Geometry: final body of the model. Coordinates: model frame, mm. A direction names the side the tool comes from. Round coordinates to 2 decimals unless told otherwise and drop trailing zeros. Order: outer loops, then holes, each group sorted by start corner. A loop starts at its lowest first (then second) coordinate and runs counter-clockwise, first axis right, second up. Notation, with made-up numbers: M 89.25,0 L 126.25,0 A22 cw 126.25,10 Z; hole C 46.25,60.25 d11. An arc over 180 degrees is marked long. Return JSON: item names as keys, results as strings. Group by question number.
Q1. Cut plane A-A on x = 25. Output: boundary loops of the cut face in (y, z).
Q2. Cut plane D-D on z = 5. Output: boundary loops of the cut face in (x, y).
Q3. Ray query, probe 1 along Y at (x, z) = (25, -0.8); probe 2 along Z at (x, y) = (6, 42.5); probe 3 along Y at (x, z) = (9.5, 5.5). Return the intervals inside material, ascending.
Q4. Mould query, pull axis Y, two halves, no side actions, for faces 3 (the face through (26.301, 24.143, -0.986)), 4 (the face through (25, 45, -1)), 5 (the face through (0, 1, 13)). Classes: released by +Y, released by -Y, zero draft, split by the parting line, or undercut.
Q5. Cut plane B-B on y = 30. Output: boundary loops of the cut face in (x, z).
Q6. Cut plane C-C on x = 44. Output: boundary loops of the cut face in (y, z), and give its area (3 significant figures).
Q7. Contact query for flat-ended pins moving along their axis: pin 1 (15 mm diameter, centred on x = 14, z = 16.5, fed in from +Y); pin 2 (1.5 mm diameter, centred on x = 41, y = 36.5, fed in from +Z). Output: stop coordinate, or through.
Q8. Access query for faces 1 (the face through (25, 23, -2)), 2 (the face through (25, 2, 25)). Directions: +Z, -Z, +X, -X, +Y, -Y. A direction counts if a zero-diameter tool reaches every point of the face in a straight line with its end or side. Return the directions, or none.
```python
from build123d import *

# Parameters (mm, degrees)
SKETCH1_W           = 50
SKETCH1_H           = 50
BOSS_EXTRUDE1_DEPTH = 2
SKETCH2_W           = 50
SKETCH2_H           = 45
SKETCH2_R           = 6
BOSS_EXTRUDE2_DEPTH = 2


with BuildPart() as part:
    # Sketch1 → Boss-Extrude1 (new body)
    with BuildSketch(Plane(origin=(0, 0, 0), x_dir=(1, 0, 0), z_dir=(0, 1, 0))):
        with Locations((25, -25)):
            Rectangle(SKETCH1_W, SKETCH1_H)
    extrude(amount=BOSS_EXTRUDE1_DEPTH)

    # Sketch2 → Boss-Extrude2 (add)
    with BuildSketch(Plane(origin=(0, 0, 0), x_dir=(-1, 0, 0), z_dir=(0, 0, -1))):
        with Locations((-25, 22.5)):
            Rectangle(SKETCH2_W, SKETCH2_H)
        with Locations((-25, 30)):
            Circle(SKETCH2_R, mode=Mode.SUBTRACT)
    extrude(amount=BOSS_EXTRUDE2_DEPTH)


solid = part.part
```
Result sheet:
{
 "1": {"outline": "M 0,-2 L 24,-2 L 24,0 L 2,0 L 2,50 L 0,50 Z; M 36,-2 L 45,-2 L 45,0 L 36,0 Z"},
 "2": {"outline": "M 0,0 L 50,0 L 50,2 L 0,2 Z"},
 "3": {"probe 1": "y = 0 to 24, 36 to 45", "probe 2": "z = -2 to 0", "probe 3": "y = 0 to 2"},
 "4": {"face 3": "undercut", "face 4": "released by +Y", "face 5": "zero draft"},
 "5": {"outline": "M 0,-2 L 19,-2 L 19,0 L 0,0 Z; M 31,-2 L 50,-2 L 50,0 L 31,0 Z"},
 "6": {"outline": "M 0,-2 L 45,-2 L 45,0 L 2,0 L 2,50 L 0,50 Z", "area": "190 mm²"},
 "7": {"pin 1": "stops at y = 2", "pin 2": "stops at z = 0"},
 "8": {"face 1": "-Z, +X, -X, +Y, -Y", "face 2": "+Z, +X, -X, +Y"}
}
